from build123d import *

# Parameters (mm, degrees)
SKETCH1_W               = 60
SKETCH1_H               = 60
BOSS_EXTRUDE1_DEPTH     = 8
SKETCH3_R               = 6.4
SKETCH3_R_2             = 6.425
SKETCH3_R_3             = 6.45
SKETCH3_R_4             = 6.475
SKETCH3_R_5             = 6.5
SKETCH3_R_6             = 6.525
SKETCH3_R_7             = 6.55
SKETCH3_R_8             = 6.575
SKETCH3_R_9             = 6.6
CUT_EXTRUDE1_DEPTH      = 1
CUT_EXTRUDE1_DEPTH_BACK = 9
CHAMFER1_SIZE           = 0.5
SKETCH4_R               = 1
CUT_EXTRUDE2_DEPTH      = 1
CUT_EXTRUDE2_DEPTH_BACK = 2


with BuildPart() as part:
    # Sketch1 → Boss-Extrude1 (new body)
    with BuildSketch(Plane(origin=(0, 0, 0), x_dir=(1, 0, 0), z_dir=(0, 1, 0))):
        Rectangle(SKETCH1_W, SKETCH1_H)
    extrude(amount=BOSS_EXTRUDE1_DEPTH)

    # Sketch3 → Cut-Extrude1 (cut, two sides)
    with BuildSketch(Plane(origin=(0, 8, 0), x_dir=(1, 0, 0), z_dir=(0, 1, 0))) as cut_extrude1_sk:
        with Locations((-18, 18)):
            Circle(SKETCH3_R)
        with Locations((0, 18)):
            Circle(SKETCH3_R_2)
        with Locations((18, 18)):
            Circle(SKETCH3_R_3)
        with Locations((-18, 0)):
            Circle(SKETCH3_R_4)
        Circle(SKETCH3_R_5)
        with Locations((18, 0)):
            Circle(SKETCH3_R_6)
        with Locations((-18, -18)):
            Circle(SKETCH3_R_7)
        with Locations((0, -18)):
            Circle(SKETCH3_R_8)
        with Locations((18, -18)):
            Circle(SKETCH3_R_9)
    extrude(amount=CUT_EXTRUDE1_DEPTH, mode=Mode.SUBTRACT)
    extrude(cut_extrude1_sk.sketch, amount=-CUT_EXTRUDE1_DEPTH_BACK, mode=Mode.SUBTRACT)

    # Chamfer1
    chamfer1_edges = [part.edges().sort_by_distance(p)[0] for p in [
        (-6.425, 8, -18),
        (11.55, 8, -18),
        (-24.475, 8, 0),
        (-6.5, 8, 0),
        (-24.55, 8, 18),
        (11.4, 8, 18),
        (-6.575, 8, 18),
        (11.475, 8, 0),
        (-24.4, 8, -18),
    ]]
    chamfer(chamfer1_edges, length=CHAMFER1_SIZE)

    # Sketch4 → Cut-Extrude2 (cut, two sides)
    with BuildSketch(Plane(origin=(0, 8, 0), x_dir=(1, 0, 0), z_dir=(0, 1, 0))) as cut_extrude2_sk:
        with Locations((-27, 27)):
            Circle(SKETCH4_R)
    extrude(amount=CUT_EXTRUDE2_DEPTH, mode=Mode.SUBTRACT)
    extrude(cut_extrude2_sk.sketch, amount=-CUT_EXTRUDE2_DEPTH_BACK, mode=Mode.SUBTRACT)


solid = part.part
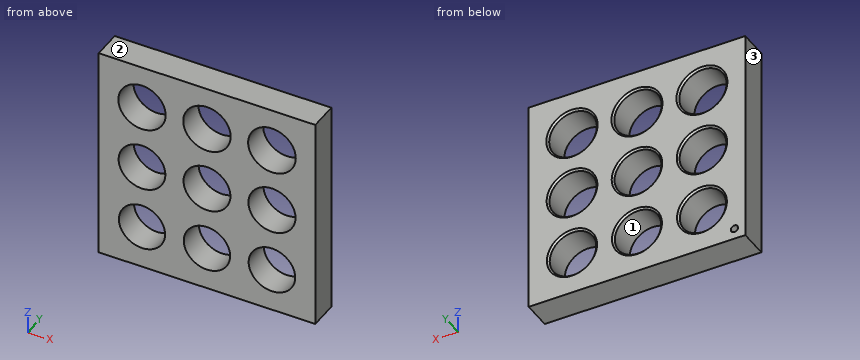
Design review of the part built by this model. Coordinates are the model's own, in mm. Face numbers are marked on the shaded views. Give positions to 0.01 mm unless a question says otherwise; leave off trailing zeros. Loops run counter-clockwise (first coordinate to the right, second up) from the corner with the lowest first, then second, coordinate; pieces in that order, holes last. Notation, with made-up numbers: (21, 38) - (59, 38) arc R19 ccw to (59, 63) - close; hole circle Ø2 at (49, -30). An arc over 180 degrees is marked (long way). Write item = value, one per line.
1) To check wall thickness, follow line 1 (Z direction, x = -18, y = 5.75) (3 decimals); line 2 (X direction, y = 2.75, z = 18) (3 decimals); line 3 (Z direction, x = 18, y = 6.25) (3 decimals). State the ranges of each line that lie inside material, in increasing order.
Result sheet:
line_1 = -30 to -24.4, -11.6 to -6.475, 6.475 to 11.45, 24.55 to 30
line_2 = -30 to -24.55, -11.45 to -6.575, 6.575 to 11.4, 24.6 to 30
line_3 = -30 to -24.45, -11.55 to -6.525, 6.525 to 11.4, 24.6 to 30
2) Take a section at A-A on x = 0. State the section outline as (y, z) points (3 decimals), and give its area (3 significant figures).
Result sheet:
outline = (0, -30) - (8, -30) - (8, -24.925) - (7.5, -24.425) - (0, -24.425) - close; (0, -11.575) - (7.5, -11.575) - (8, -11.075) - (8, -7) - (7.5, -6.5) - (0, -6.5) - close; (0, 6.5) - (7.5, 6.5) - (8, 7) - (8, 10.925) - (7.5, 11.425) - (0, 11.425) - close; (0, 24.575) - (7.5, 24.575) - (8, 25.075) - (8, 30) - (0, 30) - close
area = 167 mm2
3) Draft analysis for pull direction Z (two halves, no side actions). For the marked faces 1, 2 and 3, state which applies: +Z half, -Z half, draft (parallel to the pull), parting line (faces both ways), or undercut.
Result sheet:
face_1 = undercut
face_2 = +Z half
face_3 = draft
4) Take a section at B-B on z = 18. State the section outline as (x, y) points (3 decimals), and give its area (3 significant figures).
Result sheet:
outline = (-30, 0) - (-24.55, 0) - (-24.55, 7.5) - (-25.05, 8) - (-30, 8) - close; (-11.45, 0) - (-6.575, 0) - (-6.575, 7.5) - (-7.075, 8) - (-10.95, 8) - (-11.45, 7.5) - close; (6.575, 0) - (11.4, 0) - (11.4, 7.5) - (10.9, 8) - (7.075, 8) - (6.575, 7.5) - close; (24.6, 0) - (30, 0) - (30, 8) - (25.1, 8) - (24.6, 7.5) - close
area = 164 mm2
5) Take a section at C-C on y = 2. Count the separate pieces of the cut face and the enclosed holes in it, and give its area (3 significant figures).
Result sheet:
separate_pieces = 1
enclosed_holes = 9
area = 2,410 mm2
